Job drawing, mm, ordinate dimensions from the low corner. One solid piece. Give positions to 0.01 mm unless a question says otherwise; leave off trailing zeros. Loops run counter-clockwise (first coordinate to the right, second up) from the corner with the lowest first, then second, coordinate; pieces in that order, holes last. Notation, with made-up numbers: (-13, 89.25) -> (8, 89.25) arc R24 cw to (8, 126.25) -> close; hole circle Ø6 at (-5.75, 22). An arc over 180 degrees is marked (long way). Answer as a JSON object with one key per item and string values. Group by question number.
Q1. Band-saw the part on C-C, the plane z = 4.1. Write the cut outline in (x, y) (1 decimal), plus the area to 3 significant figures.
Q2. Drop a flat-ended pin along its axis: pin 1 (5.5 mm diameter, centred on x = 56.21, y = 8.15, fed in from +Z). Give the stop position or say it passes through.
Q3. Band-saw the part on A-A, the plane x = 6. Write the cut outline in (y, z) (1 decimal).
Q4. Band-saw the part on B-B, the plane y = 34. Write the cut outline in (x, z) (1 decimal).
Q5. Wall check: probe 1 along X at (y, z) = (8, 0.5); probe 2 along Y at (x, z) = (6, 3.5) (1 decimal); probe 3 along X at (y, z) = (6, 2.8) (1 decimal). Give the ranges that are in metal, low to high. Write a range as from..to.
Q6. Band-saw the part on D-D, the plane x = 58. Write the cut outline in (y, z), plus the area to 3 significant figures.
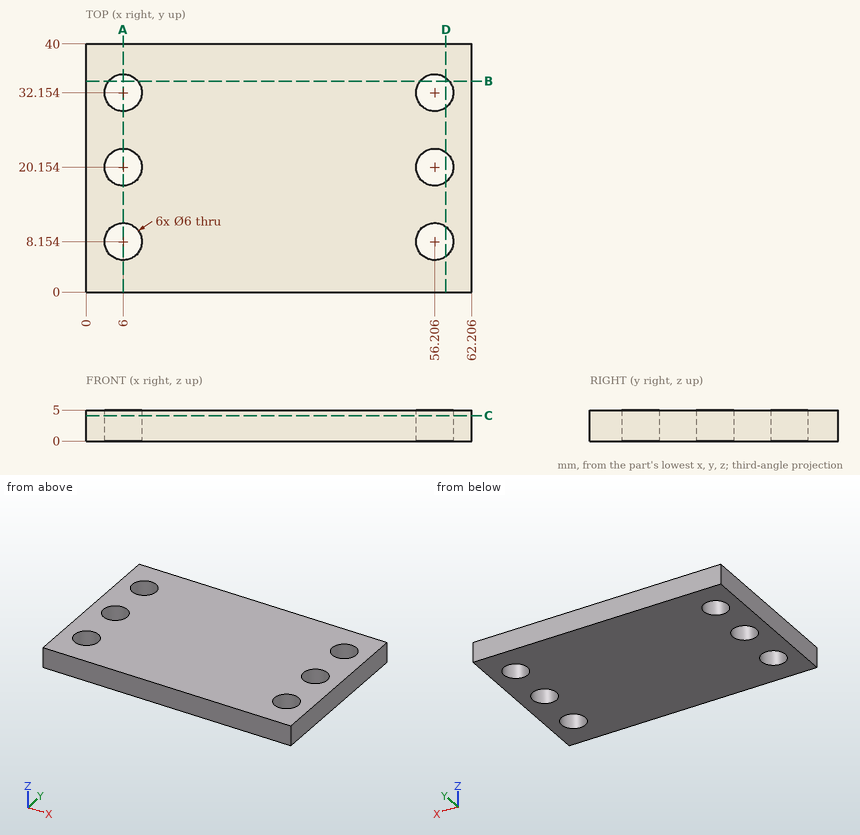
Worked answers:
{
 "1": {"outline": "(0, 0) -> (62.2, 0) -> (62.2, 40) -> (0, 40) -> close; hole circle Ø6 at (6, 8.2); hole circle Ø6 at (6, 20.2); hole circle Ø6 at (6, 32.2); hole circle Ø6 at (56.2, 8.2); hole circle Ø6 at (56.2, 20.2); hole circle Ø6 at (56.2, 32.2)", "area": "2,320 mm2"},
 "2": {"pin 1": "through"},
 "3": {"outline": "(0, 0) -> (5.2, 0) -> (5.2, 5) -> (0, 5) -> close; (11.2, 0) -> (17.2, 0) -> (17.2, 5) -> (11.2, 5) -> close; (23.2, 0) -> (29.2, 0) -> (29.2, 5) -> (23.2, 5) -> close; (35.2, 0) -> (40, 0) -> (40, 5) -> (35.2, 5) -> close"},
 "4": {"outline": "(0, 0) -> (3.6, 0) -> (3.6, 5) -> (0, 5) -> close; (8.4, 0) -> (53.8, 0) -> (53.8, 5) -> (8.4, 5) -> close; (58.6, 0) -> (62.2, 0) -> (62.2, 5) -> (58.6, 5) -> close"},
 "5": {"probe 1": "0..3, 9..53.21, 59.2..62.21", "probe 2": "0..5.2, 11.2..17.2, 23.2..29.2, 35.2..40", "probe 3": "0..3.9, 8.1..54.1, 58.3..62.2"},
 "6": {"outline": "(0, 0) -> (5.75, 0) -> (5.75, 5) -> (0, 5) -> close; (10.56, 0) -> (17.75, 0) -> (17.75, 5) -> (10.56, 5) -> close; (22.56, 0) -> (29.75, 0) -> (29.75, 5) -> (22.56, 5) -> close; (34.56, 0) -> (40, 0) -> (40, 5) -> (34.56, 5) -> close", "area": "128 mm2"}
}
